Design review of the part built by this model. Coordinates are the model's own, in mm. A direction names the side the tool comes from. Round coordinates to 2 decimals unless told otherwise and drop trailing zeros. Loops run counter-clockwise (first coordinate to the right, second up) from the corner with the lowest first, then second, coordinate; pieces in that order, holes last. Notation, with made-up numbers: M 15.5,36.5 L 50.5,36.5 A26 cw 50.5,59.5 Z; hole C 35.5,38.5 d1. An arc over 180 degrees is marked long. Use a Markdown table: item, result.
from build123d import *

# Parameters (mm, degrees)
SKETCH1_W           = 32.75
SKETCH1_H           = 19.65
BOSS_EXTRUDE1_DEPTH = 1.08
SKETCH2_W           = 1.405419427
SKETCH2_H           = 1.623501752
SKETCH2_W_2         = 1.502344905
SKETCH2_H_2         = 2.713913376
SKETCH2_W_3         = 1.623501751
SKETCH2_H_3         = 2.883532962
SKETCH2_W_4         = 3.707399523
SKETCH2_H_4         = 3.707399523
SKETCH2_W_5         = 2.762376115
SKETCH2_H_5         = 2.835070223
SKETCH2_W_6         = 4.797811147
SKETCH2_H_6         = 4.918967994
SKETCH2_W_7         = 3.852787739
SKETCH2_H_7         = 4.119332803
SKETCH2_W_8         = 1.768889968
SKETCH2_H_8         = 1.332725318
BOSS_EXTRUDE2_DEPTH = 1.6
SKETCH3_W           = 6.809014809
SKETCH3_H           = 6.978634395
SKETCH3_W_2         = 3.198540765
SKETCH3_H_2         = 1.405419426
SKETCH3_W_3         = 2.786607484
SKETCH3_W_4         = 3.077383918
SKETCH3_H_3         = 1.478113535
SKETCH3_W_5         = 3.125846656
BOSS_EXTRUDE3_DEPTH = 1.45


with BuildPart() as part:
    # Sketch1 → Boss-Extrude1 (new body)
    with BuildSketch(Plane(origin=(0, 0, 0), x_dir=(1, 0, 0), z_dir=(0, 1, 0))):
        Rectangle(SKETCH1_W, SKETCH1_H)
    extrude(amount=BOSS_EXTRUDE1_DEPTH)

    # Sketch2 → Boss-Extrude2 (add)
    with BuildSketch(Plane(origin=(0, 1.08, 0), x_dir=(1, 0, 0), z_dir=(0, 1, 0))):
        with Locations((-9.983324205, 4.737232723)):
            Rectangle(SKETCH2_W, SKETCH2_H)
        with Locations((-7.099791243, 4.749348408)):
            Rectangle(SKETCH2_W_2, SKETCH2_H_2)
        with Locations((-9.680432087, -4.44645629)):
            Rectangle(SKETCH2_W_3, SKETCH2_H_3)
        with Locations((-4.761464093, -4.85838957)):
            Rectangle(SKETCH2_W_4, SKETCH2_H_4)
        with Locations((0.290776433, -1.587154698)):
            Rectangle(SKETCH2_W_5, SKETCH2_H_5)
        with Locations((10.540645702, -4.252605335)):
            Rectangle(SKETCH2_W_6, SKETCH2_H_6)
        with Locations((10.068133998, 2.253517357)):
            Rectangle(SKETCH2_W_7, SKETCH2_H_7)
        with Locations((-7.233063774, 0.20596664)):
            Rectangle(SKETCH2_W_8, SKETCH2_H_8)
    extrude(amount=BOSS_EXTRUDE2_DEPTH)

    # Sketch3 → Boss-Extrude3 (add)
    with BuildSketch(Plane.XZ):
        with Locations((-0.860213615, 0.920792039)):
            Rectangle(SKETCH3_W, SKETCH3_H)
        with Locations((-11.049504459, -4.918967994)):
            Rectangle(SKETCH3_W_2, SKETCH3_H_2)
        with Locations((-7.596534316, -4.918967994)):
            Rectangle(SKETCH3_W_3, SKETCH3_H_2)
        with Locations((-8.178087182, 5.415711068)):
            Rectangle(SKETCH3_W_4, SKETCH3_H_3)
        with Locations((-11.691635749, 5.415711068)):
            Rectangle(SKETCH3_W_5, SKETCH3_H_3)
    extrude(amount=BOSS_EXTRUDE3_DEPTH)


solid = part.part
1. Take a section at A-A on y = -0.9. Give the boundary of the cut face in (x, z), and give its area (3 significant figures).
Check values:
| item | result |
|---|---|
| outline | M -13.25,4.68 L -10.13,4.68 L -10.13,6.15 L -13.25,6.15 Z; M -12.65,-5.62 L -9.45,-5.62 L -9.45,-4.22 L -12.65,-4.22 Z; M -9.72,4.68 L -6.64,4.68 L -6.64,6.15 L -9.72,6.15 Z; M -8.99,-5.62 L -6.2,-5.62 L -6.2,-4.22 L -8.99,-4.22 Z; M -4.26,-2.57 L 2.54,-2.57 L 2.54,4.41 L -4.26,4.41 Z |
| area | 65.1 mm² |
2. Take a section at C-C on z = 5. Give the boundary of the cut face in (x, y) (3 decimals), and give its area (3 significant figures).
Check values:
| item | result |
|---|---|
| outline | M -16.375,0 L -13.255,0 L -13.255,-1.45 L -10.129,-1.45 L -10.129,0 L -9.717,0 L -9.717,-1.45 L -6.639,-1.45 L -6.639,0 L 16.375,0 L 16.375,1.08 L 12.94,1.08 L 12.94,2.68 L 8.142,2.68 L 8.142,1.08 L -2.908,1.08 L -2.908,2.68 L -6.615,2.68 L -6.615,1.08 L -8.869,1.08 L -8.869,2.68 L -10.492,2.68 L -10.492,1.08 L -16.375,1.08 Z |
| area | 60.6 mm² |
3. Take a section at B-B on x = 10. Give the boundary of the cut face in (y, z) (3 decimals), and give its area (3 significant figures).
Check values:
| item | result |
|---|---|
| outline | M 0,-9.825 L 1.08,-9.825 L 1.08,-4.313 L 2.68,-4.313 L 2.68,-0.194 L 1.08,-0.194 L 1.08,1.793 L 2.68,1.793 L 2.68,6.712 L 1.08,6.712 L 1.08,9.825 L 0,9.825 Z |
| area | 35.7 mm² |
4. Insertion check: pin 1 (0.8 mm diameter, centred on y = 2, z = -4.5, fed in from -X); pin 2 (3 mm diameter, centred on x = 5.5, z = 3, fed in from +Y); pin 3 (0.7 mm diameter, centred on x = -7.5, y = -1, fed in from -Z). Each pin has a flat end and moves straight along its axis. Give the tip position at first contact, or say it passes through.
Check values:
| item | result |
|---|---|
| pin 1 | stops at x = -10.69 |
| pin 2 | stops at y = 1.08 |
| pin 3 | stops at z = -5.62 |
5. Take a section at D-D on y = 1.85. Count the separate pieces of the cut face and the enclosed holes in it, and give its area (3 significant figures).
Check values:
| item | result |
|---|---|
| separate pieces | 8 |
| enclosed holes | 0 |
| area | 74.4 mm² |
6. Machinability: for faces 5 (the face through (-8, -1, 4.677)), 6 (the face through (-6.203, -1, -5)), 7 (the face through (-8, -1, -5.622)), which of the approach directions +Z, -Z, +X, -X, +Y, -Y give a long, thin tool a straight path to every point of the face, cutting with its end or side? Answer none if there is none.
Check values:
| item | result |
|---|---|
| face 5 | +X, -X, -Y |
| face 6 | +Z, -Z, +X, -Y |
| face 7 | -Z, +X, -X, -Y |
7. The part is to be moulded in two halves that separate along Z. For faces 1 (the face through (11, 2, 6.712)), 2 (the face through (-10.686, 2, -5)), 3 (the face through (-12, -1, 4.677)), 4 (the face through (-1, -1, -2.569)), say which applies: pulls with the +Z half, pulls with the -Z half, needs draft (parallel to the pull), parting line crosses it, or undercut.
Check values:
| item | result |
|---|---|
| face 1 | pulls with the +Z half |
| face 2 | needs draft |
| face 3 | undercut |
| face 4 | pulls with the -Z half |
8. Wall thickness on line 1 along X through (y, z) = (1.45, 2); line 2 along Z through (x, y) = (-11, -0.2); line 3 along Z through (x, y) = (10.5, 1.9): over which ranges is each line inside the solid? List them lowest first. Write a range as from..to.
Check values:
| item | result |
|---|---|
| line 1 | x = -1.09..1.67, 8.14..12.94 |
| line 2 | z = -5.62..-4.22, 4.68..6.15 |
| line 3 | z = -4.31..-0.19, 1.79..6.71 |
